Verification items for this drawing (mm, ordinates from the low corner). Round coordinates to 2 decimals unless told otherwise and drop trailing zeros. Order: outer loops, then holes, each group sorted by start corner. A loop starts at its lowest first (then second) coordinate and runs counter-clockwise, first axis right, second up.
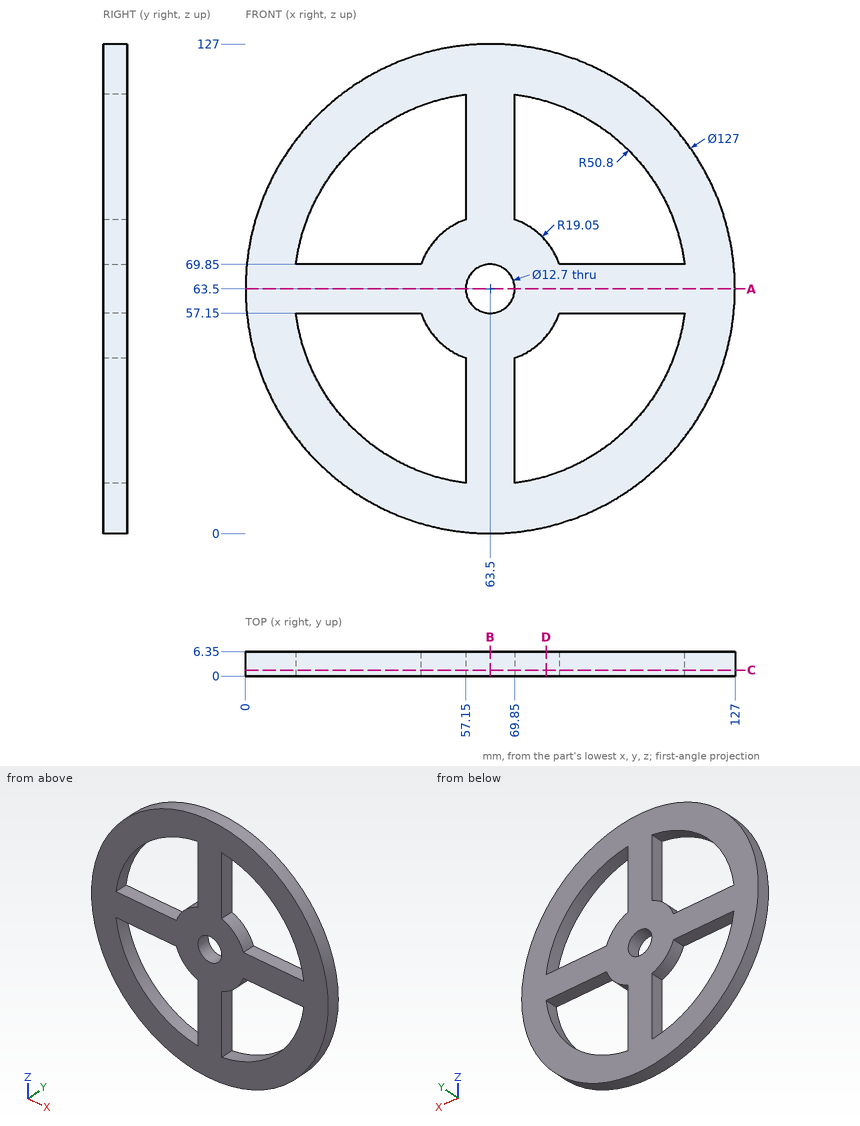
Item 1: Sectioned sample at B-B (x = 63.5). Record the cut outline in (y, z), and give its area (3 significant figures).
Answer:
outline: (0, 0) - (6.35, 0) - (6.35, 57.15) - (0, 57.15) - close; (0, 69.85) - (6.35, 69.85) - (6.35, 127) - (0, 127) - close
area: 726 mm2
Item 2: Sectioned sample at A-A (z = 63.5). Record the cut outline in (x, y).
Answer:
outline: (0, 0) - (57.15, 0) - (57.15, 6.35) - (0, 6.35) - close; (69.85, 0) - (127, 0) - (127, 6.35) - (69.85, 6.35) - close
Item 3: Scan lines: line 1 along Z through (x, y) = (63.5, 3.75); line 2 along Z through (x, y) = (84, 5.25); line 3 along Z through (x, y) = (86.5, 3.75). Record each from-to range of solid material in increasing order.
Answer:
line 1: z = 0 to 57.15, 69.85 to 127
line 2: z = 3.4 to 17.02, 57.15 to 69.85, 109.98 to 123.6
line 3: z = 4.31 to 18.2, 57.15 to 69.85, 108.8 to 122.69
Item 4: Sectioned sample at C-C (y = 1.5). Record the cut outline in (x, z).
Answer:
outline: circle Ø127 at (63.5, 63.5); hole (13.1, 57.15) arc R50.8 ccw to (57.15, 13.1) - (57.15, 45.54) arc R19.05 cw to (45.54, 57.15) - close; hole (13.1, 69.85) - (45.54, 69.85) arc R19.05 cw to (57.15, 81.46) - (57.15, 113.9) arc R50.8 ccw to start; hole circle Ø12.7 at (63.5, 63.5); hole (69.85, 13.1) arc R50.8 ccw to (113.9, 57.15) - (81.46, 57.15) arc R19.05 cw to (69.85, 45.54) - close; hole (69.85, 81.46) arc R19.05 cw to (81.46, 69.85) - (113.9, 69.85) arc R50.8 ccw to (69.85, 113.9) - close
Item 5: Sectioned sample at D-D (x = 78). Record the cut outline in (y, z).
Answer:
outline: (0, 1.68) - (6.35, 1.68) - (6.35, 14.81) - (0, 14.81) - close; (0, 51.14) - (6.35, 51.14) - (6.35, 75.86) - (0, 75.86) - close; (0, 112.19) - (6.35, 112.19) - (6.35, 125.32) - (0, 125.32) - close
Item 6: Go/stop test with flat-tipped pins: P1, Ø1.5, axis at x = 33, y = 1, coming from the -Z side; P2, Ø3, axis at y = 2.5, z = 28, coming from the +X side; P3, Ø3, axis at y = 3.5, z = 103.5, coming from the +X side. Record where each tip stops, or that it passes through.
Answer:
P1: stops at z = 7.4
P2: stops at x = 117.13
P3: stops at x = 114
